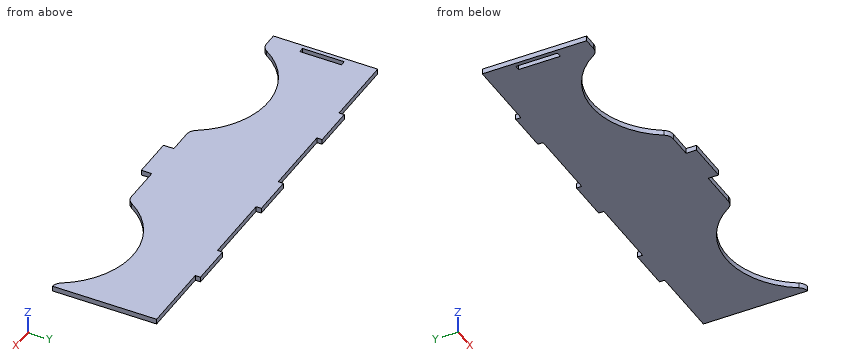
from build123d import *

# Parameters (mm, degrees)
SKETCH1_W           = 2.5
SKETCH1_H           = 20
BOSS_EXTRUDE1_DEPTH = 1.25
FILLET2_R           = 5


with BuildPart() as part:
    # Sketch1 → Boss-Extrude1 (new, symmetric)
    with BuildSketch(Plane.XY):
        with BuildLine():
            Line((-100, -25), (-100, 25))
            Line((-100, 25), (-65, 25))
            Line((-65, 25), (-65, 27.5))
            Line((-65, 27.5), (-45, 27.5))
            Line((-45, 27.5), (-45, 25))
            Line((-45, 25), (-10, 25))
            Line((-10, 25), (-10, 27.5))
            Line((-10, 27.5), (10, 27.5))
            Line((10, 27.5), (10, 25))
            Line((10, 25), (45, 25))
            Line((45, 25), (45, 27.5))
            Line((45, 27.5), (65, 27.5))
            Line((65, 27.5), (65, 25))
            Line((65, 25), (100, 25))
            Line((100, 25), (100, -25))
            Line((100, -25), (97.62, -25))
            ThreePointArc((97.62, -25), (64.453752096, -5), (31.287504193, -25))
            Line((31.287504193, -25), (10, -25))
            Line((10, -25), (10, -30))
            Line((10, -30), (-10, -30))
            Line((-10, -30), (-10, -25))
            Line((-10, -25), (-24.407504193, -25))
            ThreePointArc((-24.407504193, -25), (-57.573752096, -5), (-90.74, -25))
            Line((-90.74, -25), (-100, -25))
        make_face()
        with Locations((-96.75, 0)):
            Rectangle(SKETCH1_W, SKETCH1_H, mode=Mode.SUBTRACT)
    extrude(amount=BOSS_EXTRUDE1_DEPTH, both=True)

    # Fillet2
    # the kernel refuses this fillet: 5 mm, written as the material it takes off along each edge
    with BuildSketch(Plane(origin=(97.62, -25, 7.962737252), x_dir=(-0.49803133074323064, 0.8671590359317758, 0), z_dir=(0, 0, -1))) as fillet2_piece_1:
        with BuildLine():
            CenterArc((2.864101227, 4.996794646), FILLET2_R, 215.915482701, 52.032817446)
            Line((-1.185314567, 2.063838506), (-1.266302883, 2.005179383))
            ThreePointArc((-1.266302883, 2.005179383), (-0.679373187, 0.98211612), (-0.086715904, -0.049803133))
            Line((-0.086715904, -0.049803133), (0.003580127, -0.099935893))
            ThreePointArc((0.003580127, -0.099935893), (1.34254745, -0.075959846), (2.681514774, -0.099935893))
            Line((2.681514774, -0.099935893), (2.685094901, 0))
        make_face()
    extrude(amount=15.925474504, mode=Mode.SUBTRACT)
    with BuildSketch(Plane(origin=(31.287504193, -25, 8.473162128), x_dir=(-1, 0, 0), z_dir=(0, 0, -1))) as fillet2_piece_2:
        with BuildLine():
            CenterArc((2.889264851, 5), FILLET2_R, 211.965718751, 58.034281249)
            Line((-1.352560179, 2.352941176), (-1.437396679, 2.3))
            ThreePointArc((-1.437396679, 2.3), (-0.741683603, 1.138874159), (-0.088443328, -0.046666667))
            Line((-0.088443328, -0.046666667), (0, -0.1))
            Line((0, -0.1), (2.889264851, -0.1))
            Line((2.889264851, -0.1), (2.889264851, 0))
        make_face()
    extrude(amount=16.946324255, mode=Mode.SUBTRACT)
    with BuildSketch(Plane(origin=(-24.407504193, -25, -8.473162128), x_dir=(-0.4983656192119462, 0.8669669599168663, 0), z_dir=(0, 0, 1)), Plane(origin=(-90.74, -25, 8.473162128), x_dir=(0.4983656192119447, 0.8669669599168673, 0), z_dir=(0, 0, -1))) as fillet2_piece_3:
        with BuildLine():
            CenterArc((2.894924533, -4.99672526), FILLET2_R, 92.073789733, 58.034281249)
            Line((-1.439910267, -2.504897164), (-1.526606963, -2.455060602))
            Line((-1.526606963, -2.455060602), (-0.086696696, 0.049836562))
            Line((-0.086696696, 0.049836562), (0.003618656, 0.099934505))
            ThreePointArc((0.003618656, 0.099934505), (1.356995875, 0.075439453), (2.710373094, 0.099934505))
            Line((2.710373094, 0.099934505), (2.71399175, 0))
        make_face()
    extrude(amount=16.946324255, mode=Mode.SUBTRACT)


solid = part.part
Design review of the part built by this model. Coordinates are the model's own, in mm. Give positions to 0.01 mm unless a question says otherwise; leave off trailing zeros. Order: outer loops, then holes, each group sorted by start corner. A loop starts at its lowest first (then second) coordinate and runs counter-clockwise, first axis right, second up.
1. For pin 1 Ø1.2 at (y, z) = (26, -0.5) entering from +X; pin 2 Ø1.2 at (x, z) = (-98, 0) entering from -Y; pin 3 Ø0.8 at (y, z) = (-28, 0) entering from -X, all flat-tipped, find the tip position at first contact; note any pin that passes through.
Solution:
pin 1: stops at x = 65
pin 2: stops at y = -25
pin 3: stops at x = -10
2. To check wall thickness, follow L1, parallel to X at y = -23, z = -0.75; L2, parallel to Y at x = -26.5, z = -0.4; L3, parallel to Y at x = 23, z = 0.7. State the ranges of each line that lie inside material, in increasing order.
Solution:
L1: x = -100 to -89.63, -25.52 to 32.4, 96.51 to 100
L2: y = -21.51 to 25
L3: y = -25 to 25
3. Add section B-B, the plane x = -13. State the section outline as (y, z) points, then the cut area to 3 significant figures.
Solution:
outline: (-25, -1.25) - (25, -1.25) - (25, 1.25) - (-25, 1.25) - close
area: 125 mm2
4. Add section C-C, the plane x = -79. State the section outline as (y, z) points, then the cut area to 3 significant figures.
Solution:
outline: (-11.72, -1.25) - (25, -1.25) - (25, 1.25) - (-11.72, 1.25) - close
area: 91.8 mm2
